from build123d import *

# Parameters (mm, degrees)
BOSS_EXTRUDE2_DEPTH = 37.5
SKETCH2_W           = 80
SKETCH2_H           = 2.5
BOSS_EXTRUDE3_DEPTH = 10
SKETCH3_R           = 1.5
CUT_EXTRUDE1_DEPTH  = 10
SKETCH4_R           = 1.5
CUT_EXTRUDE2_DEPTH  = 10


with BuildPart() as part:
    # Sketch1 → Boss-Extrude2 (new body)
    with BuildSketch(Plane.XY):
        with BuildLine():
            ThreePointArc((-112.5, 0), (-97.123106012, 37.123106012), (-60, 52.5))
            Line((-60, 52.5), (60, 52.5))
            ThreePointArc((60, 52.5), (97.123106012, 37.123106012), (112.5, 0))
            Line((112.5, 0), (115, 0))
            ThreePointArc((115, 0), (98.890872965, 38.890872965), (60, 55))
            Line((60, 55), (-60, 55))
            ThreePointArc((-60, 55), (-98.890872965, 38.890872965), (-115, 0))
            Line((-115, 0), (-112.5, 0))
        make_face()
    extrude(amount=BOSS_EXTRUDE2_DEPTH)

    # Sketch2 → Boss-Extrude3 (add)
    with BuildSketch(Plane.XY.offset(37.5)):
        with Locations((0, 53.75)):
            Rectangle(SKETCH2_W, SKETCH2_H)
    extrude(amount=BOSS_EXTRUDE3_DEPTH)

    # Sketch3 → Cut-Extrude1 (cut)
    with BuildSketch(Plane(origin=(0, 55, 0), x_dir=(1, 0, 0), z_dir=(0, 1, 0))):
        with Locations(Location((-33, -41.25, 0), (0, 0, 270))):
            Circle(SKETCH3_R)
        with Locations(Location((-11, -41.25, 0), (0, 0, 270))):
            Circle(SKETCH3_R)
        with Locations(Location((11, -41.25, 0), (0, 0, 270))):
            Circle(SKETCH3_R)
        with Locations(Location((33, -41.25, 0), (0, 0, 270))):
            Circle(SKETCH3_R)
    extrude(amount=-CUT_EXTRUDE1_DEPTH, mode=Mode.SUBTRACT)

    # Sketch4 → Cut-Extrude2 (cut)
    with BuildSketch(Plane(origin=(0, 55, 0), x_dir=(1, 0, 0), z_dir=(0, 1, 0))):
        with Locations(Location((-55, -3.75, 0), (0, 0, 270))):
            Circle(SKETCH4_R)
        with Locations(Location((-33, -3.75, 0), (0, 0, 270))):
            Circle(SKETCH4_R)
        with Locations(Location((-11, -3.75, 0), (0, 0, 270))):
            Circle(SKETCH4_R)
        with Locations(Location((11, -3.75, 0), (0, 0, 270))):
            Circle(SKETCH4_R)
        with Locations(Location((33, -3.75, 0), (0, 0, 270))):
            Circle(SKETCH4_R)
        with Locations(Location((55, -3.75, 0), (0, 0, 270))):
            Circle(SKETCH4_R)
    extrude(amount=-CUT_EXTRUDE2_DEPTH, mode=Mode.SUBTRACT)


solid = part.part
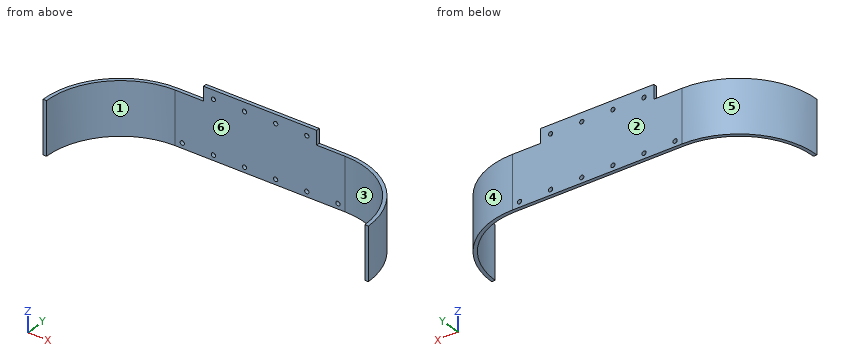
The listing builds one solid part. Answer for the finished solid, in the listing's coordinates (mm). Face numbers are marked on the shaded views. A direction names the side the tool comes from. Coordinates: 2 decimals unless noted, no trailing zeros. Write each loop counter-clockwise with the first axis right and the second up, starting at its lowest first coordinate (ties: lowest second). Pieces come first, ordered by that corner, then holes. Notation, with made-up numbers: M -4.5,-30 L 28.5,-30 A23 cw 28.5,0 Z; hole C 73.25,52 d11. An arc over 180 degrees is marked long. Write each question's results on one line, items separated by ' | '.
Item 1: Given P1, Ø1.2, axis at y = 53.5, z = 42, coming from the -X side; P2, Ø5, axis at y = 49, z = 33, coming from the -X side; P3, Ø4, axis at y = 14, z = 35.5, coming from the -X side, each flat-ended and moving along its own axis, determine where each tip first touches the part or whether it passes through.
Answer below:
P1: x = -40 | P2: x = -89.37 | P3: x = -113.67
Item 2: Consider probe 1 along X at (y, z) = (53.35, 41.25); probe 2 along Y at (x, z) = (16.5, 36.5); probe 3 along X at (y, z) = (38.5, 25). Determine where each line is inside the solid, lowest interval first. Write a range as [from, to].
Answer below:
probe 1: [-40, -34.5], [-31.5, -12.5], [-9.5, 9.5], [12.5, 31.5], [34.5, 40] | probe 2: [52.5, 55] | probe 3: [-99.28, -95.69], [95.69, 99.28]
Item 3: The part is cut by section D-D on y = 14.5. Determine the outline of the cut face in (x, z).
Answer below:
outline: M -113.05,0 L -110.46,0 L -110.46,37.5 L -113.05,37.5 Z; M 110.46,0 L 113.05,0 L 113.05,37.5 L 110.46,37.5 Z
Item 4: For a pull along X with two mould halves and no side action, classify the marked faces 3, 4, 5 and 6 as released by +X, released by -X, zero draft, split by the parting line, or undercut.
Answer below:
face 3: undercut | face 4: released by +X | face 5: released by -X | face 6: undercut
Item 5: Which of the six approach directions +Z, -Z, +X, -X, +Y, -Y give full straight-line access (tool end or side, diameter ignored) to the marked faces 1 and 2?
Answer below:
face 1: +Z, -Z, -Y | face 2: +Z, -Z, +X, -X, +Y
Item 6: The part is cut by section C-C on x = 51.5. Determine the outline of the cut face in (y, z), and give its area (4 significant figures).
Answer below:
outline: M 52.5,0 L 55,0 L 55,37.5 L 52.5,37.5 Z | area: 93.75 mm2
Item 7: The part is cut by section B-B on z = 30. Determine the outline of the cut face in (x, y), and give its area (3 significant figures).
Answer below:
outline: M -115,0 L -112.5,0 A52.5 cw -60,52.5 L 60,52.5 A52.5 cw 112.5,0 L 115,0 A55 ccw 60,55 L -60,55 A55 ccw Z | area: 722 mm2
Item 8: The part is cut by section A-A on y = 44. Determine the outline of the cut face in (x, z), and give its area (3 significant figures).
Answer below:
outline: M -93,0 L -88.64,0 L -88.64,37.5 L -93,37.5 Z; M 88.64,0 L 93,0 L 93,37.5 L 88.64,37.5 Z | area: 327 mm2
